from build123d import *

# Parameters (mm, degrees)
BOSS_EXTRUDE1_DEPTH          = 3.175
SKETCH2_R                    = 14.2875
CUT_EXTRUDE1_DEPTH           = 131.459778054
F_10_0_1935_DIAMETER_HOLE2_D = 4.9149
FILLET1_R                    = 3.175


with BuildPart() as part:
    # Sketch1 → Boss-Extrude1 (new, symmetric)
    with BuildSketch(Plane.XY):
        Polygon((-76.2, 29.162153383), (-127, -21.637846617), (127, -21.637846617), (76.2, 29.162153383), align=None)
    extrude(amount=BOSS_EXTRUDE1_DEPTH, both=True)

    # Sketch2 → Cut-Extrude1 (cut, through all)
    with BuildSketch(Plane.XY.offset(3.175)):
        with Locations((-36.107951031, -2.587846617)):
            Circle(SKETCH2_R)
    extrude(amount=-CUT_EXTRUDE1_DEPTH, mode=Mode.SUBTRACT)

    # #10 (0.1935) Diameter Hole2 (through all)
    with Locations(Plane(origin=(67.351920908, 20.049720233, 3.175), x_dir=(1, 0, 0), z_dir=(0, 0, 1))):
        with Locations((0, 0), (31.430896424, -31.430896424), (-134.703841816, 0), (-166.13473824, -31.430896424)):
            Hole(F_10_0_1935_DIAMETER_HOLE2_D / 2)

    # Fillet1
    fillet1_edges = [part.edges().sort_by_distance(p)[0] for p in [
        (76.2, 29.162153383, 0),
        (127, -21.637846617, 0),
        (-127, -21.637846617, 0),
        (-76.2, 29.162153383, 0),
    ]]
    fillet(fillet1_edges, radius=FILLET1_R)


solid = part.part
Can you work these out from the model? Positions are in its coordinate system, mm. Round coordinates to 2 decimals unless told otherwise and drop trailing zeros. Order: outer loops, then holes, each group sorted by start corner. A loop starts at its lowest first (then second) coordinate and runs counter-clockwise, first axis right, second up. Notation, with made-up numbers: (-14, 40) - (29, 40) arc R18 ccw to (29, 73) - close; hole circle Ø2 at (-2.5, 19.25). An arc over 180 degrees is marked (long way). Answer in a Markdown table with one row per item.
(1) Please list where these lines run through material, in increasing order: L1, parallel to X at y = -9.5, z = 2.25; L2, parallel to Y at x = -37, z = -2.75; L3, parallel to X at y = 7.5, z = -2.5. Write a range as from..to.
From the geometry:
| item | result |
|---|---|
| L1 | x = -114.86..-100.36, -97.2..-48.61, -23.6..97.2, 100.36..114.86 |
| L2 | y = -21.64..-16.85, 11.67..29.16 |
| L3 | x = -97.86..-46.23, -25.99..97.86 |
(2) For P1, Ø2, axis at y = -8.5, z = 0, coming from the +X side; P2, Ø5.5, axis at x = -98.78, y = -11.38, coming from the +Z side (3 decimals); P3, Ø1, axis at y = -5.5, z = -0.5, coming from the -X side; P4, Ø1, axis at y = 6, z = -2, coming from the -X side, each with a flat end and sliding along its axis, tell me the tip position at first contact or that it passes through.
From the geometry:
| item | result |
|---|---|
| P1 | stops at x = 114.86 |
| P2 | stops at z = 3.175 |
| P3 | stops at x = -111.36 |
| P4 | stops at x = -99.86 |
(3) Suppose I cut it at C-C, the plane z = -0.5. Count the separate pieces of the cut face and the enclosed holes in it, plus the area to 3 significant figures.
From the geometry:
| item | result |
|---|---|
| separate pieces | 1 |
| enclosed holes | 5 |
| area | 9,580 mm2 |
(4) Suppose I cut it at B-B, the plane x = -47.5. Please give me the cut outline in (y, z) (3 decimals).
From the geometry:
| item | result |
|---|---|
| outline | (-21.638, -3.175) - (-11.211, -3.175) - (-11.211, 3.175) - (-21.638, 3.175) - close; (6.035, -3.175) - (29.162, -3.175) - (29.162, 3.175) - (6.035, 3.175) - close |
(5) Suppose I cut it at D-D, the plane x = -80.5. Please give me the cut outline in (y, z) (3 decimals).
From the geometry:
| item | result |
|---|---|
| outline | (-21.638, -3.175) - (24.862, -3.175) - (24.862, 3.175) - (-21.638, 3.175) - close |
(6) Suppose I cut it at A-A, the plane y = 8. Please give me the cut outline in (x, z) (3 decimals), plus the area to 3 significant figures.
From the geometry:
| item | result |
|---|---|
| outline | (-97.362, -3.175) - (-45.701, -3.175) - (-45.701, 3.175) - (-97.362, 3.175) - close; (-26.515, -3.175) - (97.362, -3.175) - (97.362, 3.175) - (-26.515, 3.175) - close |
| area | 1,110 mm2 |
(7) If we mould it in two halves opening along X, with no side actions, what happens to faces 1 (the face through (-2, 4, -3.175)), 2 (the face through (65.08, 19.11, -0.04)), 3 (the face through (-122.3, -19.6, 0))? For each: released by +X, released by -X, zero draft, split by the parting line, or undercut.
From the geometry:
| item | result |
|---|---|
| face 1 | zero draft |
| face 2 | undercut |
| face 3 | released by -X |
